```python
from build123d import *

# Parameters (mm, degrees)
BOSS_EXTRUDE1_DEPTH      = 100
BOSS_EXTRUDE2_START      = 15
BOSS_EXTRUDE2_DEPTH      = 15
CUT_EXTRUDE1_DEPTH       = 15
SKETCH4_W                = 33
SKETCH4_H                = 40
CUT_EXTRUDE2_DEPTH       = 137.596313355
BOSS_EXTRUDE3_DEPTH      = 5
BOSS_EXTRUDE3_DEPTH_BACK = 10
SKETCH5_W                = 47
SKETCH5_H                = 15
BOSS_EXTRUDE4_DEPTH      = 5
BOSS_EXTRUDE4_DEPTH_BACK = 10
SKETCH6_W                = 40
SKETCH6_H                = 15


with BuildPart() as part:
    # Sketch1 → Boss-Extrude1 (new body)
    with BuildSketch(Plane.XY):
        with BuildLine():
            Line((0, 0), (-40, 0))
            Line((-40, 0), (-40, -24.764457872))
            ThreePointArc((-40, -24.764457872), (-75.554844009, 31.952220257), (-30, 81))
            Line((-30, 81), (-30, 25))
            ThreePointArc((-30, 25), (-27.071067812, 17.928932188), (-20, 15))
            Line((-20, 15), (0, 15))
            Line((0, 15), (0, 0))
        make_face()
    extrude(amount=-BOSS_EXTRUDE1_DEPTH)

    # Sketch2 → Boss-Extrude2 (add)
    with BuildSketch(Plane.XY.offset(BOSS_EXTRUDE2_START)):
        with BuildLine():
            Line((0, 0), (0, 5))
            Line((0, 5), (-75.500062866, 21.048033769))
            ThreePointArc((-75.500062866, 21.048033769), (-64.273998003, -6.913628491), (-40, -24.764457872))
            Line((-40, -24.764457872), (-40, 0))
            Line((-40, 0), (0, 0))
        make_face()
    extrude(amount=-BOSS_EXTRUDE2_DEPTH)

    # Sketch3 → Cut-Extrude1 (cut)
    with BuildSketch(Plane(origin=(0, 15, 0), x_dir=(1, 0, 0), z_dir=(0, 1, 0))):
        with BuildLine():
            Line((-5, 90), (-5, 10))
            ThreePointArc((-5, 10), (-10, 5), (-15, 10))
            Line((-15, 10), (-15, 90))
            ThreePointArc((-15, 90), (-10, 95), (-5, 90))
        make_face()
    extrude(amount=-CUT_EXTRUDE1_DEPTH, mode=Mode.SUBTRACT)

    # Sketch4 → Cut-Extrude2 (cut, through all)
    with BuildSketch(Plane(origin=(-30, 0, 0), x_dir=(0, 0, -1), z_dir=(1, 0, 0))):
        with Locations((46.5, 61)):
            Rectangle(SKETCH4_W, SKETCH4_H)
    extrude(amount=-CUT_EXTRUDE2_DEPTH, mode=Mode.SUBTRACT)

    # Sketch5 → Boss-Extrude3 (add, two sides: drawn at the far end of the back side and taken through both)
    with BuildSketch(Plane(origin=(-30, 0, 0), x_dir=(0, 0, -1), z_dir=(1, 0, 0)).offset(-BOSS_EXTRUDE3_DEPTH_BACK)):
        with Locations((86.5, 58.5)):
            Rectangle(SKETCH5_W, SKETCH5_H)
    extrude(amount=BOSS_EXTRUDE3_DEPTH + BOSS_EXTRUDE3_DEPTH_BACK)

    # Sketch6 → Boss-Extrude4 (add, two sides: drawn at the far end of the back side and taken through both)
    with BuildSketch(Plane(origin=(-30, 0, 0), x_dir=(0, 0, -1), z_dir=(1, 0, 0)).offset(-BOSS_EXTRUDE4_DEPTH_BACK)):
        with Locations((10, 58.5)):
            Rectangle(SKETCH6_W, SKETCH6_H)
    extrude(amount=BOSS_EXTRUDE4_DEPTH + BOSS_EXTRUDE4_DEPTH_BACK)


solid = part.part
```
Check sheet for the modelled part. Datum: model origin and axes. Units: mm. A direction names the side the tool comes from. Give positions to 0.01 mm unless a question says otherwise; leave off trailing zeros. Loops run counter-clockwise (first coordinate to the right, second up) from the corner with the lowest first, then second, coordinate; pieces in that order, holes last. Notation, with made-up numbers: (13, 2) - (55, 2) arc R28 ccw to (55, 37) - close; hole circle Ø9 at (70, 4.25). An arc over 180 degrees is marked (long way). One line per question, with ' | ' between items. Start each with the question number.
1. Draft check along X on faces 4 (the flat face through (-40, 59, -105)), 5 (the cylindrical face through (-10, 8, -95)), 6 (the flat face through (0, 7, -42)). Enter one of: released by +X, released by -X, zero draft, split by the parting line, or undercut.
2. Gauge pin test, flat ends, axial feed: pin 1 Ø5 at (y, z) = (61, 6.5) entering from -X; pin 2 Ø10 at (y, z) = (-6, -13.5) entering from +X; pin 3 Ø3 at (x, z) = (-35.5, -77) entering from +Y. Record the tip position at first contact, or that the pin passes through.
3. Material ranges on line 1 along Z through (x, y) = (-45.5, 73); line 2 along Z through (x, y) = (-72, 36); line 3 along Z through (x, y) = (-50.5, -0.5), recorded low to high. Write a range as [from, to].
4. Cross-section at C-C, the plane y = 43. Enter the section's corners in (x, z), plus the area to 3 significant figures.
5. Cross-section at D-D, the plane x = -42. Enter the section's corners in (y, z), plus the area to 3 significant figures.
6. Cross-section at A-A, the plane z = -34.5. Enter the section's corners in (x, y).
7. Set-up check for faces 1 (the flat face through (-30, 74, -15)), 2 (the flat face through (-40, -13, -42)), 3 (the cylindrical face through (-27.15, 18.01, -49.3)): record each of +Z, -Z, +X, -X, +Y, -Y from which the full face is reachable in a straight line by a thin tool's end or side.
8. Cross-section at B-B, the plane x = -10. Enter the section's corners in (y, z).
Check result:
1) face 4: released by -X | face 5: undercut | face 6: released by +X
2) pin 1: stops at x = -40 | pin 2: stops at x = -40 | pin 3: stops at y = 80.17
3) line 1: z = [-100, -63], [-30, 0] | line 2: z = [-100, 0] | line 3: z = [-100, 15]
4) outline: (-73.35, -100) - (-30, -100) - (-30, -63) - (-73.35, -63) - close; (-73.35, -30) - (-30, -30) - (-30, 0) - (-73.35, 0) - close | area: 2,900 mm2
5) outline: (-23.97, -100) - (77.52, -100) - (77.52, -63) - (41, -63) - (41, -30) - (77.52, -30) - (77.52, 0) - (13.93, 0) - (13.93, 15) - (-23.97, 15) - close | area: 9,510 mm2
6) outline: (-73.93, 41) arc R55 ccw to (-40, -24.76) - (-40, 0) - (-15, 0) - (-15, 15) - (-20, 15) arc R10 cw to (-30, 25) - (-30, 41) - close; (-5, 0) - (0, 0) - (0, 15) - (-5, 15) - close
7) face 1: +Z, -Z, +X, +Y | face 2: +Z, -Z, +X, -Y | face 3: +Z, -Z, +X
8) outline: (0, -100) - (15, -100) - (15, -95) - (0, -95) - close; (0, -5) - (15, -5) - (15, 0) - (7.13, 0) - (7.13, 15) - (0, 15) - close
